Check sheet for the modelled part. Datum: model origin and axes. Units: mm. A direction names the side the tool comes from. Round coordinates to 2 decimals unless told otherwise and drop trailing zeros. Order: outer loops, then holes, each group sorted by start corner. A loop starts at its lowest first (then second) coordinate and runs counter-clockwise, first axis right, second up. Notation, with made-up numbers: M 6,17 L 43,17 A26 ccw 43,45 Z; hole C 67,-37 d7. An arc over 180 degrees is marked long. One line per item, written item: value. Start each with the question number.
(1) Cross-section at B-B, the plane z = 2.25. Enter the section's corners in (x, y) (3 decimals).
(2) Thickness scan on L1, parallel to Y at x = 0, z = 7.75 (3 decimals); L2, parallel to Z at x = 4, y = 24.5. Record the ranges inside material, lowest first.
(3) Depth check by flat-ended pin: pin 1 Ø1 at (x, z) = (-11.5, 16) entering from +Y; pin 2 Ø5.5 at (y, z) = (-15, 12.5) entering from -X; pin 3 Ø1.5 at (x, z) = (-15.5, 4.5) entering from +Y. Enter the tip coordinate at first touch or a pass-through.
(4) Cross-section at A-A, the plane y = 0. Enter the section's corners in (x, z) (3 decimals), and give its area (3 significant figures).
(5) Cross-section at C-C, the plane x = 0. Enter the section's corners in (y, z) (3 decimals), and give its area (3 significant figures).
(6) Access from +Z, -Z, +X, -X, +Y, -Y to the whole of each face (thin tool, end or side, straight path). Record for faces 1 (the face through (0, 0, 18)), 2 (the face through (2.5, -21, 17)), 3 (the face through (8, 24.3, 1.5)).
from build123d import *

# Parameters (mm, degrees)
F0_R      = 32.5
F1_DEPTH  = 18
F2_R      = 3
F3_R      = 1
F4_R      = 25.405
F5_DEPTH  = 9.104
F6_R      = 27.5
F6_R_2    = 25.405
F7_DEPTH  = 1.5
F9_DEPTH  = 7
F11_DEPTH = 2


# Not quite as in the source:
# - the program builds the solid bodies; features that only make, move or delete a surface that nothing else refers to are left out


with BuildPart() as f1:
    # F0 (on Top) → F1 (new body)
    with BuildSketch(Plane.XY):
        Circle(F0_R)
    extrude(amount=F1_DEPTH)

    # F2
    f2_edges = [f1.edges().sort_by_distance(p)[0] for p in [
        (-32.5, 0, 18),
    ]]
    fillet(f2_edges, radius=F2_R)

    # F3
    f3_edges = [f1.edges().sort_by_distance(p)[0] for p in [
        (-32.5, 0, 0),
    ]]
    fillet(f3_edges, radius=F3_R)

    # F4 (on face) → F5 (cut)
    with BuildSketch(Plane(origin=(0, 0, 0), x_dir=(1, 0, 0), z_dir=(0, 0, -1))):
        Circle(F4_R)
    extrude(amount=-F5_DEPTH, mode=Mode.SUBTRACT)

    # F6 (on face) → F7 (cut)
    with BuildSketch(Plane(origin=(0, 0, 0), x_dir=(1, 0, 0), z_dir=(0, 0, -1))):
        Circle(F6_R)
        Circle(F6_R_2, mode=Mode.SUBTRACT)
    extrude(amount=-F7_DEPTH, mode=Mode.SUBTRACT)

    # F8 (on face) → F9 (cut)
    with BuildSketch(Plane.XY.offset(18)):
        with BuildLine():
            Line((1.55, -8.9630174198), (0, -8.9630174198))
            Line((0, -8.9630174198), (-1.55, -8.9630174198))
            Line((-1.55, -8.9630174198), (-1.55, -29.459251518))
            ThreePointArc((-1.55, -29.459251518), (0, -29.5), (1.55, -29.459251518))
            Line((1.55, -29.459251518), (1.55, -8.9630174198))
        make_face()
        with BuildLine():
            Line((1.55, -32.4630174198), (1.55, -29.459251518))
            ThreePointArc((1.55, -29.459251518), (0, -29.5), (-1.55, -29.459251518))
            Line((-1.55, -29.459251518), (-1.55, -32.4630174198))
            ThreePointArc((-1.55, -32.4630174198), (0, -32.5), (1.55, -32.4630174198))
        make_face()
    extrude(amount=-F9_DEPTH, mode=Mode.SUBTRACT)

    # F10 (on face) → F11 (cut)
    with BuildSketch(Plane.XY.offset(18)):
        with BuildLine():
            ThreePointArc((-2.5, -32.403703492), (-2.0252171576, -32.4368385553), (-1.55, -32.4630174198))
            ThreePointArc((-1.55, -32.4630174198), (0, -32.5), (1.55, -32.4630174198))
            ThreePointArc((1.55, -32.4630174198), (2.0252171576, -32.4368385553), (2.5, -32.403703492))
            Line((2.5, -32.403703492), (2.5, -8.903703492))
            Line((2.5, -8.903703492), (-2.5, -8.903703492))
            Line((-2.5, -8.903703492), (-2.5, -32.403703492))
        make_face()
    extrude(amount=-F11_DEPTH, mode=Mode.SUBTRACT)


solid = f1.part
Values found:
1. outline: C 0,0 d65; hole C 0,0 d50.81
2. L1: -32.5 to -25.405, 25.405 to 32.5
2. L2: 9.1 to 18
3. pin 1: y = 30.46
3. pin 2: x = -30.1
3. pin 3: y = 28.96
4. outline: M -32.5,1 A1 ccw -31.5,0 L -27.5,0 L -27.5,1.5 L -25.405,1.5 L -25.405,9.104 L 25.405,9.104 L 25.405,1.5 L 27.5,1.5 L 27.5,0 L 31.5,0 A1 ccw 32.5,1 L 32.5,15 A3 ccw 29.5,18 L -29.5,18 A3 ccw -32.5,15 Z
4. area: 697 mm^2
5. outline: M -32.5,1 A1 ccw -31.5,0 L -27.5,0 L -27.5,1.5 L -25.405,1.5 L -25.405,9.104 L 25.405,9.104 L 25.405,1.5 L 27.5,1.5 L 27.5,0 L 31.5,0 A1 ccw 32.5,1 L 32.5,15 A3 ccw 29.5,18 L -8.904,18 L -8.904,16 L -8.963,16 L -8.963,11 L -32.5,11 Z
5. area: 534 mm^2
6. face 1: +Z, +X, -X, +Y, -Y
6. face 2: +Z, -Y
6. face 3: -Z
